Can you work these out from the model? Positions are in its coordinate system, mm. Face numbers are marked on the shaded views. A direction names the side the tool comes from. Give positions to 0.01 mm unless a question says otherwise; leave off trailing zeros. Loops run counter-clockwise (first coordinate to the right, second up) from the corner with the lowest first, then second, coordinate; pieces in that order, holes last. Notation, with made-up numbers: (21, -35.75) - (27, -35.75) arc R22 cw to (27, -17.75) - close; hole circle Ø11 at (55.25, 80). An arc over 180 degrees is marked (long way). Answer as a JSON object with one key per item and string values.
```python
from build123d import *

# Parameters (mm, degrees)
F3_DEPTH      = 20.001
F3_DEPTH_BACK = 20.001
F4_R          = 7.5
F5_DEPTH      = 21
F7_R          = 6
F8_DEPTH      = 2
F8_DEPTH_BACK = 9
F9_SIZE       = 0.5


with BuildPart() as f1:
    # F0 (on Front) → F1 (revolve)
    with BuildSketch(Plane.XZ):
        with BuildLine():
            Line((20, 0), (0, 0))
            Line((0, 0), (0, -45))
            ThreePointArc((0, -45), (14.1421356237, -39.1421356237), (20, -25))
            Line((20, -25), (20, 0))
        make_face()
    revolve(axis=Axis((0, 0, 4.3592059342), (0, 0, 1)))

    # F2 (on Front) → F3 (cut, two sides)
    with BuildSketch(Plane.XZ) as f3_sk:
        Polygon((0, -45), (12, -45), (12, -5), (0, -5), (-12, -5), (-12, -45), align=None)
    extrude(amount=-F3_DEPTH, mode=Mode.SUBTRACT)
    extrude(f3_sk.sketch, amount=F3_DEPTH_BACK, mode=Mode.SUBTRACT)

    # F4 (on Right) → F5 (join, through all)
    with BuildSketch(Plane.YZ):
        with Locations((0, -25)):
            Circle(F4_R)
    extrude(amount=F5_DEPTH)

    # F6: F1 across plane


with BuildPart() as f1_1:
    add(f1.part)
    add(f1.part.mirror(Plane.YZ))

    # F7 (on face) → F8 (join, two sides)
    with BuildSketch(Plane.YZ.offset(21)) as f8_sk:
        with Locations((0, -25)):
            Circle(F7_R)
    extrude(amount=F8_DEPTH)
    extrude(f8_sk.sketch, amount=-F8_DEPTH_BACK)

    # F9
    f9_edges = [f1_1.edges().sort_by_distance(p)[0] for p in [
        (23, -6, -25),
        (-21, -7.5, -25),
        (21, -7.5, -25),
    ]]
    chamfer(f9_edges, length=F9_SIZE)


solid = f1_1.part
```
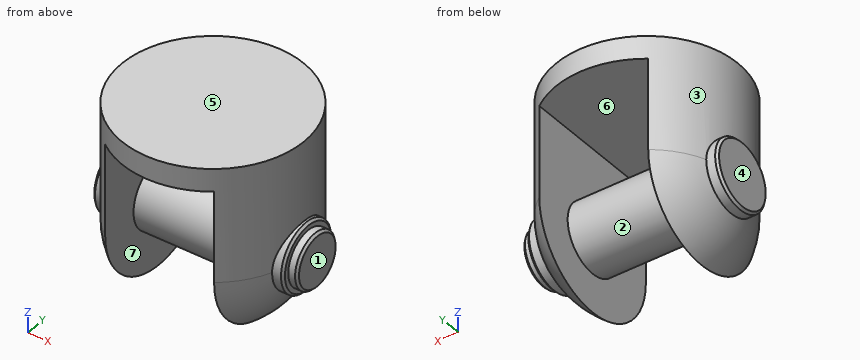
1) I'm going to push flat-ended pins straight in: P1, Ø12, axis at x = 1, y = -8.5, coming from the -Z side; P2, Ø6, axis at x = -8, z = -28, coming from the +Y side; P3, Ø10, axis at x = 0, z = -20, coming from the -Y side. Where does each tip first touch, or does it pass through?
Check sheet entries:
{"P1": "z = -32.07", "P2": "y = 7.5", "P3": "y = -7.5"}
2) If we mould it in two halves opening along Z, with no side actions, what happens to the marked faces 4, 5, 6 and 7? For each: released by +Z, released by -Z, zero draft, split by the parting line, or undercut.
Check sheet entries:
{"face 4": "zero draft", "face 5": "released by +Z", "face 6": "undercut", "face 7": "undercut"}
3) Imagine slicing it at D-D on z = -37.5. Write out the boundary of the cut face in (x, y).
Check sheet entries:
{"outline": "(-12, -9.99) - (-12, 9.99) arc R15.61 ccw to start; (12, -9.99) arc R15.61 ccw to (12, 9.99) - close"}
4) Which directions (+Z, -Z, +X, -X, +Y, -Y) give clear straight access to the entire face, cutting with the end or side of a thin tool? Please do the marked faces 1, 2 and 3.
Check sheet entries:
{"face 1": "+Z, -Z, +X, +Y, -Y", "face 2": "none", "face 3": "+Z"}
5) Imagine slicing it at B-B on x = 0. Write out the boundary of the cut face in (y, z).
Check sheet entries:
{"outline": "(-20, -5) - (20, -5) - (20, 0) - (-20, 0) - close; circle Ø15 at (0, -25)"}
6) I need wall thicknesses on L1, parallel to Z at x = -0.5, y = 8; L2, parallel to X at y = -3, z = -37.5; L3, parallel to X at y = -12.5, z = -28.5. Which ranges of each line are inside material? Lowest first, please.
Check sheet entries:
{"L1": "-5 to 0", "L2": "-15.32 to -12, 12 to 15.32", "L3": "-15.22 to -12, 12 to 15.22"}
7) Imagine slicing it at A-A on y = 0. Write out the boundary of the cut face in (x, z), and give its area (3 significant figures).
Check sheet entries:
{"outline": "(-21, -32) - (-20.5, -32.5) - (-18.54, -32.5) arc R20 ccw to (-12, -41) - (-12, -32.5) - (12, -32.5) - (12, -41) arc R20 ccw to (18.54, -32.5) - (20.5, -32.5) - (21, -32) - (21, -31) - (22.5, -31) - (23, -30.5) - (23, -19.5) - (22.5, -19) - (21, -19) - (21, -18) - (20.5, -17.5) - (20, -17.5) - (20, 0) - (-20, 0) - (-20, -17.5) - (-20.5, -17.5) - (-21, -18) - close; hole (-12, -17.5) - (12, -17.5) - (12, -5) - (-12, -5) - close", "area": "1,120 mm2"}
8) Imagine slicing it at C-C on x = 8.5. Write out the boundary of the cut face in (y, z), and give its area (3 significant figures).
Check sheet entries:
{"outline": "(-18.1, -5) - (18.1, -5) - (18.1, 0) - (-18.1, 0) - close; circle Ø15 at (0, -25)", "area": "358 mm2"}
